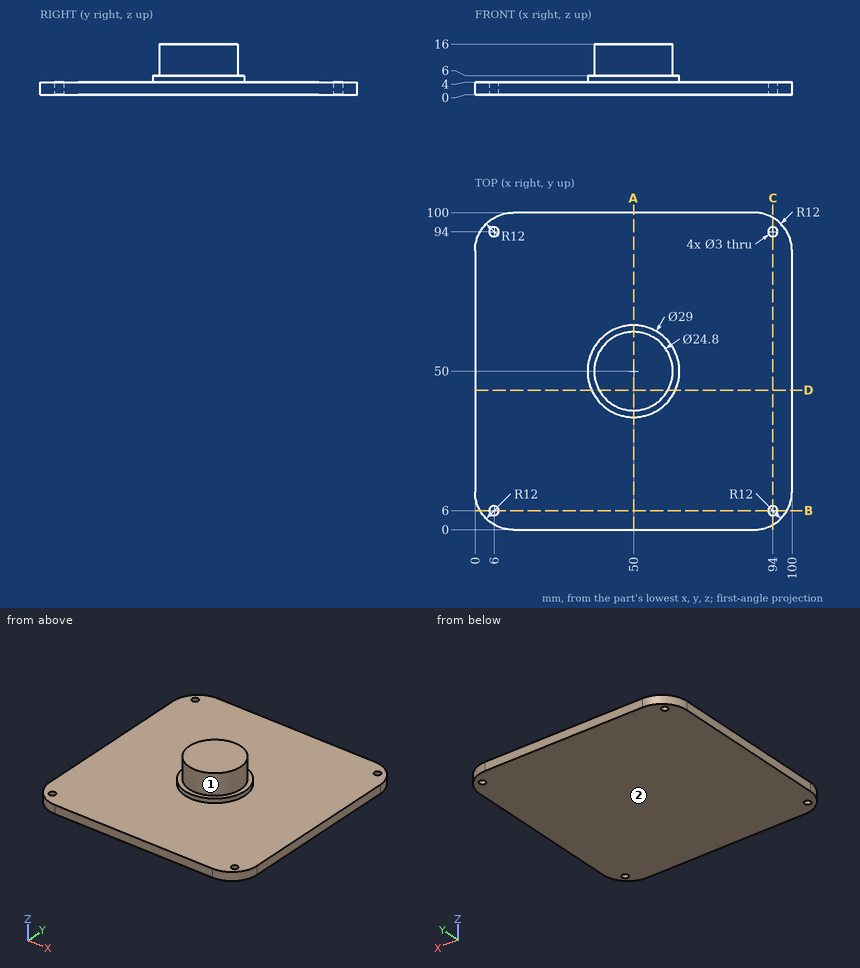
Here's the drawing with two shaded views (mm, measured from the low corner). I have some questions. A direction names the side the tool comes from. Give positions to 0.01 mm unless a question says otherwise; leave off trailing zeros. Write each loop counter-clockwise with the first axis right and the second up, starting at its lowest first coordinate (ties: lowest second). Pieces come first, ordered by that corner, then holes. Notation, with made-up numbers: (43, 75) -> (63, 75) arc R17 cw to (63, 89) -> close; hole circle Ø3 at (-8.5, -25). An arc over 180 degrees is marked (long way). Use one line per item in the form item = value.
1) Suppose I cut it at D-D (y = 44). Please give me the cut outline in (x, z).
Verdict:
outline = (0, 0) -> (100, 0) -> (100, 4) -> (63.2, 4) -> (63.2, 6) -> (60.85, 6) -> (60.85, 16) -> (39.15, 16) -> (39.15, 6) -> (36.8, 6) -> (36.8, 4) -> (0, 4) -> close
2) I'm going to push flat-ended pins straight in: pin 1 (10 mm diameter, centred on x = 34, y = 11.5, fed in from -Z); pin 2 (2.5 mm diameter, centred on x = 94, y = 6, fed in from -Z); pin 3 (3 mm diameter, centred on x = 56, y = 33.5, fed in from +Z). Where does each tip first touch, or does it pass through?
Verdict:
pin_1 = 0
pin_2 = through
pin_3 = 4
3) Suppose I cut it at B-B (y = 6). Please give me the cut outline in (x, z).
Verdict:
outline = (1.61, 0) -> (4.5, 0) -> (4.5, 4) -> (1.61, 4) -> close; (7.5, 0) -> (92.5, 0) -> (92.5, 4) -> (7.5, 4) -> close; (95.5, 0) -> (98.39, 0) -> (98.39, 4) -> (95.5, 4) -> close
4) On a 3-axis mill with a long thin cutter (end or side, diameter ignored), from which of +Z, -Z, +X, -X, +Y, -Y can I reach the whole of each face in a straight line? I mean the marked faces 1 and 2. Say none if no direction works.
Verdict:
face_1 = +Z
face_2 = -Z, +X, -X, +Y, -Y
5) Suppose I cut it at A-A (x = 50). Please give me the cut outline in (y, z), and give its area (3 significant figures).
Verdict:
outline = (0, 0) -> (100, 0) -> (100, 4) -> (64.5, 4) -> (64.5, 6) -> (62.4, 6) -> (62.4, 16) -> (37.6, 16) -> (37.6, 6) -> (35.5, 6) -> (35.5, 4) -> (0, 4) -> close
area = 706 mm2
6) If I drill on L1, parallel to Y at x = 94, z = 2.75; L2, parallel to Z at x = 69.5, y = 71.5; L3, parallel to X at y = 50.5, z = 15, over which ranges is the centre line in solid material (lowest first)? Write a range as [from, to].
Verdict:
L1 = [1.61, 4.5], [7.5, 92.5], [95.5, 98.39]
L2 = [0, 4]
L3 = [37.61, 62.39]
